Autodesk Inventor part; units mm, degrees
ref_plane "YZ Plane" through (0, 0, 0) normal (1, 0, 0) x (0, 1, 0)
ref_plane "XZ Plane" through (0, 0, 0) normal (0, 1, 0) x (-1, 0, 0)
ref_plane "XY Plane" through (0, 0, 0) normal (0, 0, 1) x (1, 0, 0)
sketch "Sketch1" plane through (0, 0, 0) normal (0, 0, 1) x (1, 0, 0)
  line L0 (0, 0) -> (-12.7, 0) construction
  line L1 (-12.7, 0) -> (-12.7, 53.975) construction
  line L2 (-12.7, 53.975) -> (0, 53.975) construction
  line L3 (0, 53.975) -> (0, 0) construction
  line L4 (-12.7, 53.975) -> (-25.4, 53.975) construction
  line L5 (-12.7, 53.975) -> (0, 53.975) construction
  line L6 (-25.4, 53.975) -> (-25.4, 0) construction
  line L7 (-25.4, 0) -> (-12.7, 0) construction
  circle A0 centre (-12.7, 6.35) radius 6.35 construction
  circle A1 centre (-12.7, 47.625) radius 6.35 construction
  line L8 (-12.7, 47.625) -> (-18.1993, 50.8) construction
  line L9 (-12.7, 47.625) -> (-6.35, 47.625) construction
  line L10 (-12.7, 47.625) -> (-7.2007, 50.8) construction
  line L11 (-12.7, 47.625) -> (-6.35, 47.625) construction
  line L12 (0, 0) -> (-25.4, 0)
  line L13 (0, 0) -> (0, -1.5875)
  line L14 (0, 0) -> (1.5875, 0) construction
  line L15 (0, -1.5875) -> (-26.9875, -1.5875)
  arc A2 (-7.2007, 50.8) -> (-18.1993, 50.8) centre (-12.7, 47.625) ccw
  line L16 (-7.2007, 50.8) -> (0, 38.328)
  line L17 (-7.2007, 50.8) -> (7.2007, 50.8) construction
  line L18 (-18.1993, 50.8) -> (-24.5493, 39.8015)
  line L19 (-18.1993, 50.8) -> (-5.4993, 50.8) construction
  line L20 (-25.4, 0) -> (-25.4, 36.6265)
  line L21 (-19.5741, 51.5937) -> (-26.1368, 40.2268)
  line L22 (-26.9875, -1.5875) -> (-26.9875, 37.0518)
  arc A3 (-26.1368, 40.2268) -> (-26.9875, 37.0518) centre (-20.6375, 37.0518) ccw
  arc A4 (-24.5493, 39.8015) -> (-25.4, 36.6265) centre (-19.05, 36.6265) ccw
  line L23 (-5.8259, 51.5937) -> (1.3748, 39.1217)
  arc A5 (-5.8259, 51.5937) -> (-19.5741, 51.5937) centre (-12.7, 47.625) ccw
  arc A6 (0, 38.328) -> (1.3748, 39.1217) centre (0.6874, 38.7248) ccw
  point P0 (-25.4, 38.328)
  dimension "d0" = 12.7
  dimension "d1" = 53.975
  dimension "d2" = 12.7
  dimension "d3" = 180
  dimension "d4" = 53.975
  dimension "d5" = 90
  dimension "d6" = 12.7
  dimension "d7" = 12.7
  dimension "d8" = 6.35
  dimension "d9" = 6.35
  dimension "d10" = 6.35
  dimension "d11" = 150
  dimension "d12" = 6.35
  dimension "d13" = 30
  dimension "d14" = 1.5875
  dimension "d15" = 90
  dimension "d16" = 26.9875
  dimension "d17" = 6.35
  dimension "d18" = 60
  dimension "d19" = 120
  dimension "d20" = 90
  dimension "d21" = 1.5875
  dimension "d22" = 6.35
  dimension "d23" = 6.35
  dimension "d24" = 1.5875
  dimension "d25" = 7.9375
  dimension "d26" = 0
extrude "Extrusion1" add sketch "Sketch1" along normal blind 1524
sketch "Sketch2" plane through (-26.9875, -1.5875, 0) normal (-1, 0, 0) x (0, 0, 1)
  line L0 (0, 38.6393) -> (0, 0)
  line L1 (0, 0) -> (1524, 0)
  line L2 (1524, 38.6393) -> (1524, 0)
  line L3 (0, 38.6393) -> (1524, 38.6393)
  point P0 (0, 1.5875)
  point P1 (1498.6, 19.05)
  dimension "d29" = 19.05
  dimension "d30" = 25.4
hole "Hole1" at (-26.9875, 17.4625, 1498.6) direction (1, 0, 0) diameter 9.525 end through all
sketch "Sketch3" plane through (-26.9875, -1.5875, 0) normal (-1, 0, 0) x (0, 0, 1)
  circle A0 centre (1498.6, 19.05) radius 4.7625
  line L0 (0, 38.6393) -> (0, 0)
  line L1 (0, 0) -> (1524, 0)
  line L2 (1524, 38.6393) -> (1524, 0)
  line L3 (0, 38.6393) -> (1524, 38.6393)
  circle A1 centre (31.75, 19.05) radius 4.7625
  line L4 (15.875, 28.575) -> (15.875, 25.4) construction
  line L5 (15.875, 28.575) -> (15.875, 31.75) construction
  line L6 (12.7, 28.575) -> (12.7, 31.75) construction
  line L7 (12.7, 28.575) -> (12.7, 25.4) construction
  line L8 (15.875, 12.7) -> (15.875, 15.875) construction
  line L9 (12.7, 12.7) -> (12.7, 15.875) construction
  line L10 (15.875, 12.7) -> (15.875, 9.525) construction
  line L11 (12.7, 12.7) -> (12.7, 9.525) construction
  arc A2 (15.875, 25.4) -> (15.875, 31.75) centre (15.875, 28.575) ccw
  arc A3 (12.7, 31.75) -> (12.7, 25.4) centre (12.7, 28.575) ccw
  arc A4 (15.875, 9.525) -> (15.875, 15.875) centre (15.875, 12.7) ccw
  arc A5 (12.7, 15.875) -> (12.7, 9.525) centre (12.7, 12.7) ccw
  line L12 (15.875, 31.75) -> (12.7, 31.75)
  line L13 (15.875, 25.4) -> (12.7, 25.4)
  line L14 (15.875, 15.875) -> (12.7, 15.875)
  line L15 (15.875, 9.525) -> (12.7, 9.525)
  point P0 (0, 1.5875)
  dimension "d45" = 12.7
  dimension "d46" = 15.875
  dimension "d47" = 31.75
  dimension "d48" = 12.7
  dimension "d49" = 15.875
  dimension "d50" = 9.525
  dimension "d51" = 19.05
  dimension "d52" = 12.7
  dimension "d53" = 12.7
  dimension "d54" = 28.575
  dimension "d55" = 28.575
  dimension "d56" = 3.175
  dimension "d57" = 3.175
  dimension "d58" = 3.175
  dimension "d59" = 3.175
  dimension "d60" = 3.175
  dimension "d61" = 3.175
  dimension "d62" = 3.175
  dimension "d63" = 3.175
  dimension "d64" = 3.175
  dimension "d65" = 3.175
  dimension "d66" = 3.175
  dimension "d67" = 3.175
extrude "Extrusion2" cut sketch "Sketch3" against normal blind 25.4 contours A1 | L13 A3 L12 A2 | L15 A5 L14 A4
sketch "Sketch4" plane through (-26.9875, -1.5875, 0) normal (-1, 0, 0) x (0, 0, 1)
  line L0 (12.7, 15.875) -> (15.875, 15.875)
  arc A0 (15.875, 9.525) -> (15.875, 15.875) centre (15.875, 12.7) ccw
  line L1 (15.875, 9.525) -> (12.7, 9.525)
  arc A1 (12.7, 15.875) -> (12.7, 9.525) centre (12.7, 12.7) ccw
  line L2 (12.7, 31.75) -> (15.875, 31.75)
  arc A2 (15.875, 25.4) -> (15.875, 31.75) centre (15.875, 28.575) ccw
  line L3 (15.875, 25.4) -> (12.7, 25.4)
  arc A3 (12.7, 31.75) -> (12.7, 25.4) centre (12.7, 28.575) ccw
  circle A4 centre (31.75, 19.05) radius 4.7625
  circle A5 centre (1498.6, 19.05) radius 4.7625
  line L4 (0, 38.6393) -> (0, 0)
  line L5 (0, 0) -> (1524, 0)
  line L6 (1524, 38.6393) -> (1524, 0)
  line L7 (0, 38.6393) -> (1524, 38.6393)
  point P0 (0, 1.5875)
  point P1 (101.6, 25.9393)
  point P2 (88.9, 12.7)
  point P3 (76.2, 25.9393)
  point P4 (63.5, 12.7)
  dimension "d70" = 63.5
  dimension "d71" = 76.2
  dimension "d72" = 88.9
  dimension "d73" = 101.6
  dimension "d74" = 12.7
  dimension "d75" = 12.7
  dimension "d76" = 12.7
  dimension "d77" = 12.7
hole "Hole2" at (-26.9875, 24.3518, 101.6) at (-26.9875, 11.1125, 88.9) at (-26.9875, 24.3518, 76.2) at (-26.9875, 11.1125, 63.5) direction (1, 0, 0) diameter 6.35 end through all
sketch "Sketch5" plane through (-26.9875, -1.5875, 0) normal (-1, 0, 0) x (0, 0, 1)
  circle A0 centre (76.2, 25.9393) radius 3.175
  circle A1 centre (101.6, 25.9393) radius 3.175
  circle A2 centre (88.9, 12.7) radius 3.175
  circle A3 centre (63.5, 12.7) radius 3.175
  line L0 (12.7, 15.875) -> (15.875, 15.875)
  arc A4 (15.875, 9.525) -> (15.875, 15.875) centre (15.875, 12.7) ccw
  line L1 (15.875, 9.525) -> (12.7, 9.525)
  arc A5 (12.7, 15.875) -> (12.7, 9.525) centre (12.7, 12.7) ccw
  line L2 (12.7, 31.75) -> (15.875, 31.75)
  arc A6 (15.875, 25.4) -> (15.875, 31.75) centre (15.875, 28.575) ccw
  line L3 (15.875, 25.4) -> (12.7, 25.4)
  arc A7 (12.7, 31.75) -> (12.7, 25.4) centre (12.7, 28.575) ccw
  circle A8 centre (31.75, 19.05) radius 4.7625
  circle A9 centre (1498.6, 19.05) radius 4.7625
  line L4 (0, 38.6393) -> (0, 0)
  line L5 (0, 0) -> (1524, 0)
  line L6 (1524, 38.6393) -> (1524, 0)
  line L7 (0, 38.6393) -> (1524, 38.6393)
  point P0 (0, 1.5875)
  point P1 (706.4375, 12.7)
  point P2 (782.6375, 12.7)
  point P3 (744.5375, 12.7)
  dimension "d85" = 12.7
  dimension "d86" = 12.7
  dimension "d87" = 12.7
  dimension "d88" = 706.4375
  dimension "d89" = 744.5375
  dimension "d90" = 782.6375
hole "Hole3" at (-26.9875, 11.1125, 706.4375) at (-26.9875, 11.1125, 782.6375) at (-26.9875, 11.1125, 744.5375) direction (1, 0, 0) diameter 3.9688 end through all
properties part number "2in rail right"
Here's how the part is built. I have some questions about the finished solid (model axes, mm). Give positions to 0.01 mm unless a question says otherwise; leave off trailing zeros. Loops run counter-clockwise (first coordinate to the right, second up) from the corner with the lowest first, then second, coordinate; pieces in that order, holes last. Notation, with made-up numbers: M 51,-38 L 69,-38 A9 ccw 69,-23 Z; hole C 31.5,-17 d6. An arc over 180 degrees is marked long. Put each result on its own line as item: value. Start each with the question number.
(1) I need wall thicknesses on line 1 along Y through (x, z) = (-17.5, 1312); line 2 along Y through (x, z) = (-14.5, 641); line 3 along X through (y, z) = (47.5, 1258). Which ranges of each line are inside material? Lowest first, please. Write a range as [from, to].
(2) If we mould it in two halves opening along Y, with no side actions, what happens to faces 1 (the flat face through (-13, 0, 751)), 2 (the flat face through (-26.5, 22.9, 0)), 3 (the flat face through (-13, -1.588, 751)), 4 (the flat face through (-25.4, 18, 751))? For each: +Y half, -Y half, draft (parallel to the pull), parting line (faces both ways), or undercut.
(3) I want a section at A-A on z = 876. Please give me the cut outline in (x, y) (1 decimal).
(4) Will these pins go through, and if not, where does the flat tip stop? pin 1 Ø1.3 at (x, z) = (-26.5, 14.5) entering from +Y; pin 2 Ø8.5 at (y, z) = (11.11, 63.5) entering from -X; pin 3 Ø0.5 at (x, z) = (-26.5, 14) entering from +Y; pin 4 Ø7.5 at (y, z) = (17.46, 31.75) entering from +X.
Answer block:
1. line 1: [-1.59, 0], [51.78, 53.95]
1. line 2: [-1.59, 0], [53.71, 55.36]
1. line 3: [-21.94, -20.1], [-5.3, -3.46]
2. face 1: undercut
2. face 2: draft
2. face 3: -Y half
2. face 4: undercut
3. outline: M -27,-1.6 L 0,-1.6 L 0,0 L -25.4,0 L -25.4,36.6 A6.3 cw -24.5,39.8 L -18.2,50.8 A6.4 cw -7.2,50.8 L 0,38.3 A0.8 ccw 1.4,39.1 L -5.8,51.6 A7.9 ccw -19.6,51.6 L -26.1,40.2 A6.3 ccw -27,37.1 Z
4. pin 1: y = 40.72
4. pin 2: x = -26.99
4. pin 3: y = 40.02
4. pin 4: through
